Source: CAD feature listing. Evaluate the final solid. Frame: model axes, mm. Round coordinates to 2 decimals unless told otherwise and drop trailing zeros. Loops run counter-clockwise (first coordinate to the right, second up) from the corner with the lowest first, then second, coordinate; pieces in that order, holes last. Notation, with made-up numbers: (48, -18.75) -> (59, -18.75) arc R31 ccw to (59, 18.25) -> close; hole circle Ø4 at (-30.5, -21). An arc over 180 degrees is marked (long way). Return JSON: item names as keys, results as strings. Group by question number.
```python
from build123d import *

# Parameters (mm, degrees)
ESBO_O1_W                = 48
ESBO_O1_H                = 26
ESBO_O1_R                = 1.5
ESBO_O1_R_2              = 1
ESBO_O1_R_3              = 6.5
RESSALTO_EXTRUS_O1_DEPTH = 3
ESBO_O7_W                = 48
ESBO_O7_H                = 3
RESSALTO_EXTRUS_O4_DEPTH = 24
ESBO_O8_R                = 1
ESBO_O8_R_2              = 1.5
CORTE_EXTRUS_O2_DEPTH    = 3
CHANFRO2_SIZE            = 2


with BuildPart() as part:
    # Esboço1 → Ressalto-extrusão1 (new body)
    with BuildSketch(Plane.XY):
        Rectangle(ESBO_O1_W, ESBO_O1_H)
        with Locations((20, 0)):
            Circle(ESBO_O1_R, mode=Mode.SUBTRACT)
        with Locations((15, 8.5)):
            Circle(ESBO_O1_R_2, mode=Mode.SUBTRACT)
        with Locations((7.5, 8)):
            Circle(ESBO_O1_R, mode=Mode.SUBTRACT)
        with Locations(Location((15, -8.5, 0), (0, 0, 180))):
            Circle(ESBO_O1_R_2, mode=Mode.SUBTRACT)
        with Locations(Location((7.5, -8, 0), (0, 0, 180))):
            Circle(ESBO_O1_R, mode=Mode.SUBTRACT)
        with Locations(Location((-15, 8.5, 0), (0, 0, 180))):
            Circle(ESBO_O1_R_2, mode=Mode.SUBTRACT)
        with Locations((-7.5, -8)):
            Circle(ESBO_O1_R, mode=Mode.SUBTRACT)
        with Locations((-15, -8.5)):
            Circle(ESBO_O1_R_2, mode=Mode.SUBTRACT)
        with Locations(Location((-7.5, 8, 0), (0, 0, 180))):
            Circle(ESBO_O1_R, mode=Mode.SUBTRACT)
        with Locations(Location((-20, 0, 0), (0, 0, 180))):
            Circle(ESBO_O1_R, mode=Mode.SUBTRACT)
        with Locations((0, -4)):
            Circle(ESBO_O1_R_3, mode=Mode.SUBTRACT)
    extrude(amount=RESSALTO_EXTRUS_O1_DEPTH)

    # Esboço7 → Ressalto-extrusão4 (add)
    with BuildSketch(Plane(origin=(0, 13, 0), x_dir=(1, 0, 0), z_dir=(0, 1, 0))):
        with Locations((0, -1.5)):
            Rectangle(ESBO_O7_W, ESBO_O7_H)
    extrude(amount=RESSALTO_EXTRUS_O4_DEPTH)

    # Esboço8 → Corte-extrusão2 (cut)
    with BuildSketch(Plane.XY.offset(3)):
        with Locations((-15, 25.5)):
            Circle(ESBO_O8_R)
        with Locations((-20, 33)):
            Circle(ESBO_O8_R_2)
        with Locations((20, 33)):
            Circle(ESBO_O8_R_2)
        with Locations((15, 25.5)):
            Circle(ESBO_O8_R)
    extrude(amount=-CORTE_EXTRUS_O2_DEPTH, mode=Mode.SUBTRACT)

    # Chanfro2
    chanfro2_edges = [part.edges().sort_by_distance(p)[0] for p in [
        (-24, 37, 1.5),
        (24, 37, 1.5),
        (24, -13, 1.5),
        (-24, -13, 1.5),
    ]]
    chamfer(chanfro2_edges, length=CHANFRO2_SIZE)


solid = part.part
```
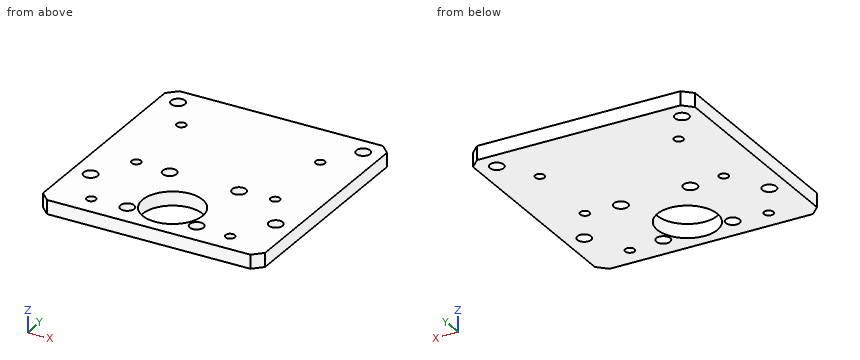
(1) Cut plane D-D (x = 0). Return loops of the section in (y, z), and give its area (3 significant figures).
(2) Cut plane A-A (x = -15). Return loops of the section in (y, z), and give its area (3 significant figures).
(3) Ray query, line 1 (Y direction, x = 15, z = 2.2); line 2 (X direction, y = -7, z = 1.6); line 3 (Y direction, x = 14.5, z = 0.4). Return the intervals inside material, ascending.
(4) Cut plane B-B (z = 1.65). Count the separate pieces of the cut face and the enclosed holes in it, and give its area (3 significant figures).
(5) Cut plane C-C (x = 7.5). Return loops of the section in (y, z), and give its area (3 significant figures).
Answers follow:
{
 "1": {"outline": "(-13, 0) -> (-10.5, 0) -> (-10.5, 3) -> (-13, 3) -> close; (2.5, 0) -> (37, 0) -> (37, 3) -> (2.5, 3) -> close", "area": "111 mm^2"},
 "2": {"outline": "(-13, 0) -> (-9.5, 0) -> (-9.5, 3) -> (-13, 3) -> close; (-7.5, 0) -> (7.5, 0) -> (7.5, 3) -> (-7.5, 3) -> close; (9.5, 0) -> (24.5, 0) -> (24.5, 3) -> (9.5, 3) -> close; (26.5, 0) -> (37, 0) -> (37, 3) -> (26.5, 3) -> close", "area": "132 mm^2"},
 "3": {"line 1": "-13 to -9.5, -7.5 to 7.5, 9.5 to 24.5, 26.5 to 37", "line 2": "-24 to -8.62, -6.38 to -5.77, 5.77 to 6.38, 8.62 to 24", "line 3": "-13 to -9.37, -7.63 to 7.63, 9.37 to 24.63, 26.37 to 37"},
 "4": {"separate pieces": "1", "enclosed holes": "15", "area": "2,180 mm^2"},
 "5": {"outline": "(-13, 0) -> (-9.5, 0) -> (-9.5, 3) -> (-13, 3) -> close; (-6.5, 0) -> (6.5, 0) -> (6.5, 3) -> (-6.5, 3) -> close; (9.5, 0) -> (37, 0) -> (37, 3) -> (9.5, 3) -> close", "area": "132 mm^2"}
}
